Verification items for the finished model (mm, model axes). A direction names the side the tool comes from. Give positions to 0.01 mm unless a question says otherwise; leave off trailing zeros. Write each loop counter-clockwise with the first axis right and the second up, starting at its lowest first coordinate (ties: lowest second). Pieces come first, ordered by that corner, then holes. Notation, with made-up numbers: (-16.75, 43.25) - (3.25, 43.25) arc R4 ccw to (3.25, 47.25) - close; hole circle Ø7 at (62, 79.25). An arc over 180 degrees is marked (long way). Put each result on its own line as item: value.
from build123d import *

# Parameters (mm, degrees)
CLINCHCUT_START    = -0.75
CLINCHCUT_DEPTH    = 0.75
CLINCHCUTPAT_COUNT = 24
CLINCHCUTPAT_ANGLE = 345
HEXCUT_DEPTH       = 0.0254


with BuildPart() as part:
    # BodySke → Body (revolve)
    with BuildSketch(Plane.XY, mode=Mode.PRIVATE) as body_sk:
        Polygon((3.78575, -1.071611123), (3.78575, -0.75), (4.45, -0.75), (4.45, 0), (3.75, 0), (3.75, 3), (3.485509529, 4.5), (2.1, 4.5), (2.1, -1.5), (3.985, -1.5), (3.985, -1.125), align=None)
    revolve(body_sk.sketch.rotate(Axis((0, -1.125, 0), (0, 1, 0)), 90), axis=Axis((0, -1.125, 0), (0, 1, 0)))

    # EndChamferSke → EndChamfer (revolve, cut)
    with BuildSketch(Plane.XY, mode=Mode.PRIVATE) as endchamfer_sk:
        Polygon((2.5, -1.754), (2.5, -1.49746), (2.1, -1.217481014), (2.1, -1.754), align=None)
        Polygon((2.5, 4.49746), (2.5, 4.754), (2.1, 4.754), (2.1, 4.217481014), align=None)
    revolve(endchamfer_sk.sketch.rotate(Axis((0, -2.54, 0), (0, 1, 0)), 90), axis=Axis((0, -2.54, 0), (0, 1, 0)), mode=Mode.SUBTRACT)

    # CliRinCutSke → ClinchCut (cut)
    with BuildSketch(Plane.XZ.offset(0.75).offset(CLINCHCUT_START)):
        with BuildLine():
            Line((0.580841555, 4.411929633), (0, 4.094))
            Line((0, 4.094), (-0.580841555, 4.411929633))
            ThreePointArc((-0.580841555, 4.411929633), (0, 4.45), (0.580841555, 4.411929633))
        make_face()
    clinchcut = extrude(amount=CLINCHCUT_DEPTH, mode=Mode.SUBTRACT)

    # ClinchCutPat: ClinchCut ×24 about axis
    clinchcutpat_axis = Axis((0, 0, 0), (0, 1, 0))
    for i in range(1, CLINCHCUTPAT_COUNT):
        add(clinchcut.rotate(clinchcutpat_axis, i * CLINCHCUTPAT_ANGLE / (CLINCHCUTPAT_COUNT - 1)), mode=Mode.SUBTRACT)

    # HexCutSke → HexCut (cut)
    with BuildSketch(Plane(origin=(0, 4.5, 0), x_dir=(-1, 0, 0), z_dir=(0, 1, 0))):
        Polygon((-1.732050808, 3), (1.732050808, 3), (3.464101615, 0), (1.732050808, -3), (-1.732050808, -3), (-3.464101615, 0), align=None)
    extrude(amount=-HEXCUT_DEPTH, mode=Mode.SUBTRACT)


solid = part.part
Q1. Scan lines: line 1 along Y through (x, z) = (2.5, -1); line 2 along X through (y, z) = (0.55, 0); line 3 along X through (y, z) = (0.9, 1.5). Record each from-to range of solid material in increasing order.
Answers follow:
line 1: y = -1.5 to 4.47
line 2: x = -3.75 to -2.1, 2.1 to 3.75
line 3: x = -3.44 to -1.47, 1.47 to 3.44
Q2. Release check for a two-part mould opening along Z. For faces 1 (the face through (-0.631, 1.462, -2.003)), 2 (the face through (2.6, 4.5, -1.8)), 3 (the face through (-3.16, 1.52, -2.02)) record: released by +Z, released by -Z, zero draft, split by the parting line, or undercut.
Answers follow:
face 1: undercut
face 2: zero draft
face 3: split by the parting line
Q3. Go/stop test with flat-tipped pins: pin 1 Ø4 at (x, z) = (0, 0) entering from +Y; pin 2 Ø1.5 at (x, y) = (-2.5, 2.5) entering from +Z. Record where each tip stops, or that it passes through.
Answers follow:
pin 1: passes through
pin 2: stops at z = 3.32
Q4. Section check A-A, the plane y = 1.45. Record the cut outline in (x, z), plus the area to 3 significant figures.
Answers follow:
outline: circle Ø7.5 at (0, 0); hole circle Ø4.2 at (0, 0)
area: 30.3 mm2
Q5. Set-up check for faces 4 (the face through (-1.2, -1.3, -3.8)), 5 (the face through (-1.14, -0.91, -3.61)), 6 (the face through (2, -1.5, -2)), 7 (the face through (2, 4.475, -2)): record each of +Z, -Z, +X, -X, +Y, -Y from which the full face is reachable in a straight line by a thin tool's end or side.
Answers follow:
face 4: -Y
face 5: none
face 6: +Z, -Z, +X, -X, -Y
face 7: +Y
